Work out the finished part from the listing and answer in its coordinate system (mm). A direction names the side the tool comes from. Coordinates: 2 decimals unless noted, no trailing zeros. Order: outer loops, then holes, each group sorted by start corner. A loop starts at its lowest first (then second) coordinate and runs counter-clockwise, first axis right, second up.
1. Flat-ended cylindrical pins translate along their axes: pin 1 Ø10 at (x, y) = (-4.5, -5.5) entering from +Z; pin 2 Ø1 at (y, z) = (8.5, 2) entering from +X; pin 3 Ø1.5 at (x, z) = (-2.5, 3) entering from +Y. Find the tip coordinate at first contact, or state that the pin passes through.
2. The part is cut by section A-A, the plane y = -7. Give the vertices of the cut face in (x, z).
3. A tool of negligible diameter and unlimited length cuts with its end or side. For faces 5 (the flat face through (8.5, 3, 2)), 6 (the flat face through (-7, 3, 2)), 7 (the flat face through (0, -11.5, 2)), from which of +Z, -Z, +X, -X, +Y, -Y can it reach the whole face along a straight path? Write none if from no direction.
4. Find the intervals of material crossed by probe 1 along Z at (x, y) = (-9.5, 7); probe 2 along X at (y, z) = (7.5, 1.8); probe 3 along X at (y, z) = (-4, 3.6), in increasing order.
5. The part is cut by section C-C, the plane z = 0.45. Give the vertices of the cut face in (x, y), then the cut area to 3 significant figures.
6. Determine the mould class of faces 1 (the flat face through (0, -12, 3.25)), 2 (the flat face through (0, -12, 1.25)), 3 (the flat face through (0, -11, 0)), 4 (the flat face through (0, -17, 1)) for opening direction Z: +Z half, -Z half, draft (parallel to the pull), parting line (faces both ways), or undercut.
7. The part is cut by section D-D, the plane x = -7.75. Give the vertices of the cut face in (y, z), then the cut area to 3 significant figures.
8. The part is cut by section B-B, the plane x = 9. Give the vertices of the cut face in (y, z).
```python
from build123d import *

# Parameters (mm, degrees)
F1_DEPTH = 4.5
F2_W     = 34
F2_H     = 2
F3_DEPTH = 5.5
F4_W     = 34
F4_H     = 2
F5_DEPTH = 5.5
F6_W     = 17
F6_H     = 2
F7_DEPTH = 5.5


with BuildPart() as f1:
    # F0 (on Top) → F1 (new body)
    with BuildSketch(Plane.XY):
        Polygon((-14, -17), (14, -17), (14, 17), (7, 17), (7, -10), (-7, -10), (-7, 17), (-14, 17), align=None)
    extrude(amount=F1_DEPTH)

    # F2 (on face) → F3 (cut)
    with BuildSketch(Plane(origin=(-14, 0, 0), x_dir=(0, -1, 0), z_dir=(-1, 0, 0))):
        with Locations((0, 2.25)):
            Rectangle(F2_W, F2_H)
    extrude(amount=-F3_DEPTH, mode=Mode.SUBTRACT)

    # F4 (on face) → F5 (cut)
    with BuildSketch(Plane.YZ.offset(14)):
        with Locations((0, 2.25)):
            Rectangle(F4_W, F4_H)
    extrude(amount=-F5_DEPTH, mode=Mode.SUBTRACT)

    # F6 (on face) → F7 (cut)
    with BuildSketch(Plane.XZ.offset(17)):
        with Locations((0, 2.25)):
            Rectangle(F6_W, F6_H)
    extrude(amount=-F7_DEPTH, mode=Mode.SUBTRACT)


solid = f1.part
```
Geometry says:
1. pin 1: stops at z = 4.5
1. pin 2: stops at x = 8.5
1. pin 3: stops at y = -10
2. outline: (-14, 0) - (-7, 0) - (-7, 4.5) - (-14, 4.5) - (-14, 3.25) - (-8.5, 3.25) - (-8.5, 1.25) - (-14, 1.25) - close; (7, 0) - (14, 0) - (14, 1.25) - (8.5, 1.25) - (8.5, 3.25) - (14, 3.25) - (14, 4.5) - (7, 4.5) - close
3. face 5: +X, +Y, -Y
3. face 6: +Z, -Z, +Y
3. face 7: +X, -X, -Y
4. probe 1: z = 0 to 1.25, 3.25 to 4.5
4. probe 2: x = -8.5 to -7, 7 to 8.5
4. probe 3: x = -14 to -7, 7 to 14
5. outline: (-14, -17) - (14, -17) - (14, 17) - (7, 17) - (7, -10) - (-7, -10) - (-7, 17) - (-14, 17) - close
5. area: 574 mm2
6. face 1: undercut
6. face 2: undercut
6. face 3: -Z half
6. face 4: draft
7. outline: (-17, 0) - (17, 0) - (17, 4.5) - (-17, 4.5) - (-17, 3.25) - (-11.5, 3.25) - (-11.5, 1.25) - (-17, 1.25) - close
7. area: 142 mm2
8. outline: (-17, 0) - (17, 0) - (17, 1.25) - (-17, 1.25) - close; (-17, 3.25) - (17, 3.25) - (17, 4.5) - (-17, 4.5) - close
